Here's the drawing with two shaded views (mm, measured from the low corner). I have some questions. Coordinates: 2 decimals unless noted, no trailing zeros. Write each loop counter-clockwise with the first axis right and the second up, starting at its lowest first coordinate (ties: lowest second). Pieces come first, ordered by that corner, then holes.
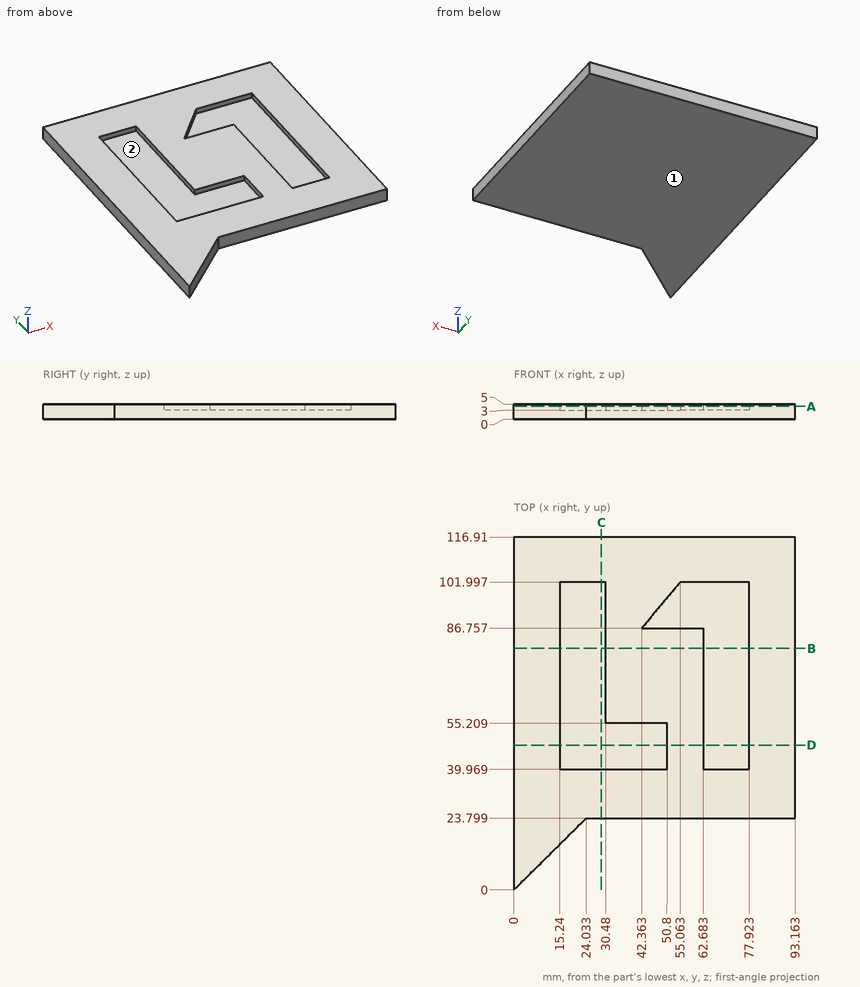
1. If we section it at A-A, the plane z = 4.2: List the corners of the cut face in (x, y) for me, plus the area to 3 significant figures.
2. If I drill on L1, parallel to X at y = 62.5, z = 4.05; L2, parallel to Y at x = 77, z = 3.6; L3, parallel to X at y = 95, z = 3.1 (1 decimal), over which ranges is the centre line in solid material (lowest first)?
3. I'm going to push flat-ended pins straight in: P1, Ø1.6, axis at x = 21.5, z = 4, coming from the -Y side; P2, Ø1.6, axis at x = 67.5, z = 4.5, coming from the -Y side. Where does each tip first touch, or does it pass through?
4. If we section it at C-C, the plane x = 29: List the corners of the cut face in (y, z) for me.
5. We'd pull the mould along X, two halves only. Please class the marked faces 1 and 2: released by +X, released by -X, zero draft, split by the parting line, or undercut.
6. If we section it at B-B, the plane y = 80: List the corners of the cut face in (x, z) for me.
7. If we section it at D-D, the plane y = 48: List the corners of the cut face in (x, z) for me, plus the area to 3 significant figures.
Answers:
1. outline: (0, 0) - (24.03, 23.8) - (93.16, 23.8) - (93.16, 116.91) - (0, 116.91) - close; hole (15.24, 39.97) - (50.8, 39.97) - (50.8, 55.21) - (30.48, 55.21) - (30.48, 102) - (15.24, 102) - close; hole (42.36, 86.76) - (62.68, 86.76) - (62.68, 39.97) - (77.92, 39.97) - (77.92, 102) - (55.06, 102) - close
1. area: 6,550 mm2
2. L1: x = 0 to 15.24, 30.48 to 62.68, 77.92 to 93.16
2. L2: y = 23.8 to 39.97, 102 to 116.91
2. L3: x = 0 to 15.2, 30.5 to 49.2, 77.9 to 93.2
3. P1: stops at y = 20.5
3. P2: stops at y = 23.8
4. outline: (23.8, 0) - (116.91, 0) - (116.91, 5) - (102, 5) - (102, 3) - (39.97, 3) - (39.97, 5) - (23.8, 5) - close
5. face 1: zero draft
5. face 2: undercut
6. outline: (0, 0) - (93.16, 0) - (93.16, 5) - (77.92, 5) - (77.92, 3) - (62.68, 3) - (62.68, 5) - (30.48, 5) - (30.48, 3) - (15.24, 3) - (15.24, 5) - (0, 5) - close
7. outline: (0, 0) - (93.16, 0) - (93.16, 5) - (77.92, 5) - (77.92, 3) - (62.68, 3) - (62.68, 5) - (50.8, 5) - (50.8, 3) - (15.24, 3) - (15.24, 5) - (0, 5) - close
7. area: 364 mm2
